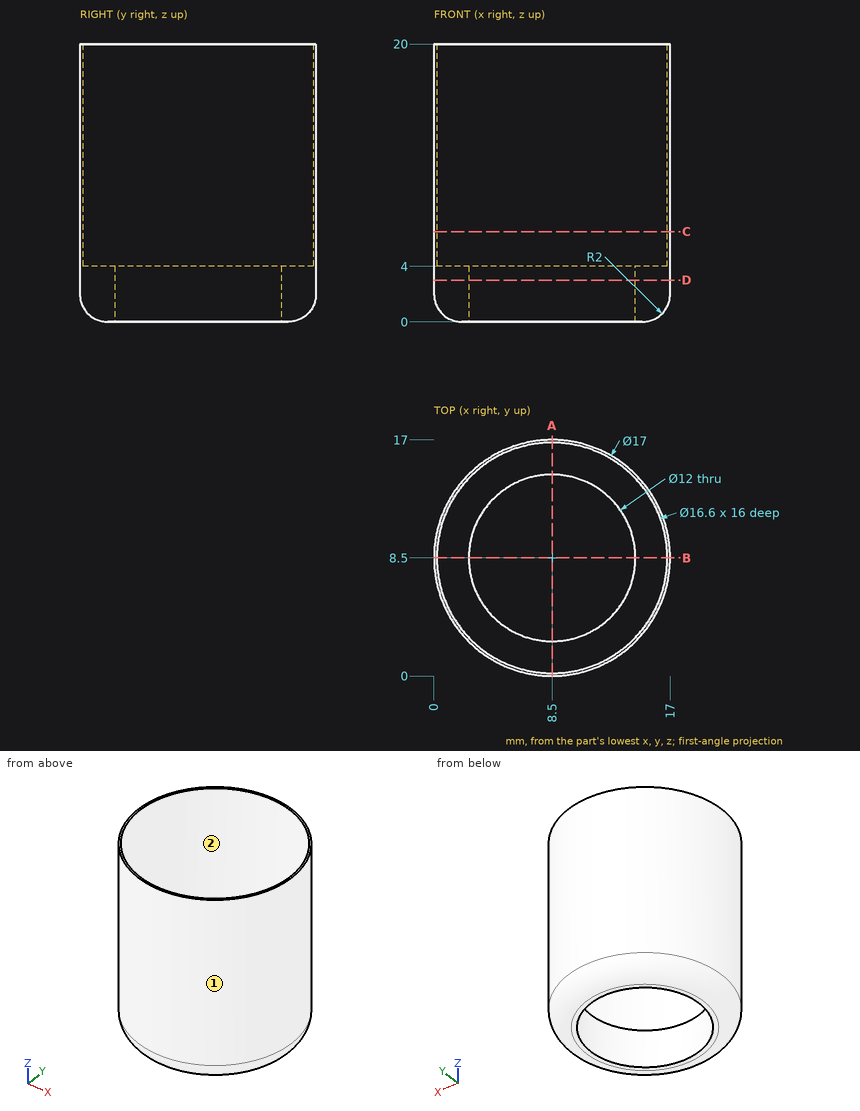
Print and shaded views of the part. All mm, measured from the part's lowest x, y and z. Give positions to 0.01 mm unless a question says otherwise; leave off trailing zeros. Write each loop counter-clockwise with the first axis right and the second up, starting at its lowest first coordinate (ties: lowest second). Pieces come first, ordered by that corner, then holes. Notation, with made-up numbers: (36.25, 54.25) - (78.25, 54.25) arc R26 cw to (78.25, 82.25) - close; hole circle Ø5 at (66, 46). An arc over 180 degrees is marked (long way). One line per question, with ' | ' between items. Start each with the question number.
(1) Two-plate mould, pull along X, no slides. Class the marked faces 1 and 2: +X half, -X half, draft (parallel to the pull), parting line (faces both ways), or undercut.
(2) Slice it at C-C on z = 6.5. Write the cut outline in (x, y), plus the area to 3 significant figures.
(3) Wall check: line 1 along Y through (x, z) = (8.5, 7.5); line 2 along Y through (x, z) = (8.5, 2.25); line 3 along Z through (x, y) = (3.75, 12.25). Give the ranges that are in metal, low to high. Write a range as from..to.
(4) Slice it at A-A on x = 8.5. Write the cut outline in (y, z).
(5) Pin check, flat tips, straight feed: P1, Ø3, axis at x = 11, z = 15.5, coming from the +Y side; P2, Ø2, axis at y = 11, z = 7, coming from the +X side; P3, Ø10, axis at x = 8.5, y = 5.5, coming from the +Z side. Stop position of each tip, or through.
(6) Slice it at D-D on z = 3. Write the cut outline in (x, y), plus the area to 3 significant figures.
Results below:
1) face 1: parting line | face 2: undercut
2) outline: circle Ø17 at (8.5, 8.5); hole circle Ø16.6 at (8.5, 8.5) | area: 10.6 mm^2
3) line 1: 0..0.2, 16.8..17 | line 2: 0..2.5, 14.5..17 | line 3: 0..4
4) outline: (0, 2) arc R2 ccw to (2, 0) - (2.5, 0) - (2.5, 4) - (0.2, 4) - (0.2, 20) - (0, 20) - close; (14.5, 0) - (15, 0) arc R2 ccw to (17, 2) - (17, 20) - (16.8, 20) - (16.8, 4) - (14.5, 4) - close
5) P1: y = 16.94 | P2: x = 16.87 | P3: z = 4
6) outline: circle Ø17 at (8.5, 8.5); hole circle Ø12 at (8.5, 8.5) | area: 114 mm^2
